For this review, take the finished solid that the model builds, in its own axes (mm). Face numbers are marked on the shaded views. A direction names the side the tool comes from. Coordinates: 2 decimals unless noted, no trailing zeros. Write each loop counter-clockwise with the first axis right and the second up, starting at its lowest first coordinate (ties: lowest second). Pieces come first, ordered by that corner, then holes. Notation, with made-up numbers: M 55,58.25 L 109,58.25 A17 ccw 109,85.25 Z; hole C 21.25,-29 d9. An arc over 180 degrees is marked long. Return JSON: item names as keys, results as strings.
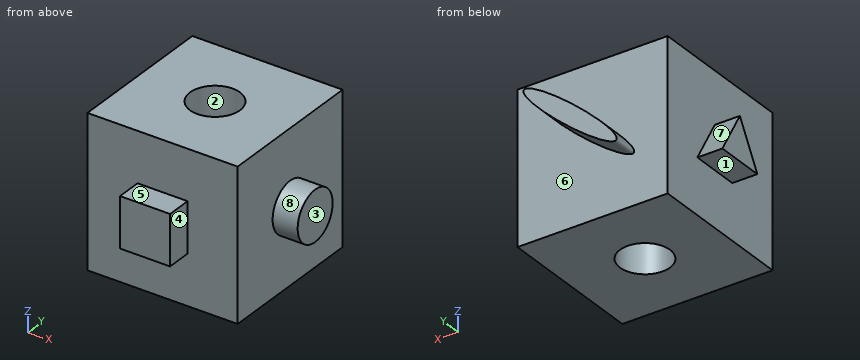
```python
from build123d import *

# Parameters (mm, degrees)
F0_W      = 76.2
F0_H      = 76.2
F1_DEPTH  = 76.2
F2_W      = 25.4
F2_H      = 25.4
F3_DEPTH  = 12.7
F4_R      = 12.7
F5_DEPTH  = 12.7
F7_D      = 25.4
F9_DEPTH  = 12.7
F11_DEPTH = 12.7


with BuildPart() as f1:
    # F0 (on Front) → F1 (new body)
    with BuildSketch(Plane.XZ):
        with Locations((-25.095452, 28.064179)):
            Rectangle(F0_W, F0_H)
    extrude(amount=F1_DEPTH)

    # F2 (on face) → F3 (join)
    with BuildSketch(Plane.XZ.offset(76.2)):
        with Locations((-25.095452, 28.064179)):
            Rectangle(F2_W, F2_H)
    extrude(amount=F3_DEPTH)

    # F4 (on face) → F5 (join)
    with BuildSketch(Plane.YZ.offset(13.004548)):
        with Locations((-38.1, 28.064179)):
            Circle(F4_R)
    extrude(amount=F5_DEPTH)

    # F7 (through all)
    with Locations(Plane.XY.offset(66.164179)):
        with Locations((-25.095452, -38.1)):
            Hole(F7_D / 2)

    # F8 (on face) → F9 (join)
    with BuildSketch(Plane(origin=(-63.195452, 0, 0), x_dir=(0, -1, 0), z_dir=(-1, 0, 0))):
        Polygon((46.956852, 17.904179), (34.256852, 39.901224), (21.556852, 17.904179), align=None)
    extrude(amount=F9_DEPTH)

    # F10 (on face) → F11 (join)
    with BuildSketch(Plane(origin=(0, 0, 0), x_dir=(-1, 0, 0), z_dir=(0, 1, 0))):
        with BuildLine():
            add(Edge.make_bspline(
                [(-0.974158, 55.745363), (-6.054851, 49.801911), (31.750569, 22.627692), (69.555988, -4.546527), (36.831261, 28.571144), (4.106534, 61.688816), (-0.974158, 55.745363)],
                knots=[0, 0, 0, 2.094395, 2.094395, 4.18879, 4.18879, 6.283185, 6.283185, 6.283185], degree=2, weights=[1, 0.5, 1, 0.5, 1, 0.5, 1]))
        make_face()
    extrude(amount=F11_DEPTH)


solid = f1.part
```
1. For the marked faces 4, 5, 6, 7 and 8, list the 3-axis set-ups (+Z, -Z, +X, -X, +Y, -Y) from which the entire face can be reached by the end or side of a thin tool; tool diameter is ignored.
Checks:
{"face 4": "+Z, -Z, +X, -Y", "face 5": "+Z, +X, -X, -Y", "face 6": "+Y", "face 7": "+Z, -X, +Y", "face 8": "+X"}
2. Clearance check with flat-ended pins moving along their axes: pin 1 Ø2 at (y, z) = (-8, 39) entering from +X; pin 2 Ø6.5 at (x, y) = (-19.5, -83.5) entering from -Z; pin 3 Ø10 at (x, y) = (-68.5, -35) entering from -Z. State where each tip first meets the part, or that it passes through.
Checks:
{"pin 1": "x = 13", "pin 2": "z = 15.36", "pin 3": "z = 17.9"}
3. Wall thickness on L1, parallel to X at y = -38, z = 8; L2, parallel to X at y = -1, z = -6; L3, parallel to Y at x = -26, z = 58.5: over which ranges is each line inside the solid? List them lowest first. Write a range as from..to.
Checks:
{"L1": "-63.2..-37.8, -12.4..13", "L2": "-63.2..13", "L3": "-76.2..-50.77, -25.43..0"}
4. We need section D-D (y = -73.5). State the section outline as (x, z) points, plus the area to 3 significant figures.
Checks:
{"outline": "M -63.2,-10.04 L 13,-10.04 L 13,66.16 L -63.2,66.16 Z", "area": "5,810 mm2"}
5. Draft analysis for pull direction X (two halves, no side actions). For the marked faces 1, 2 and 3, state which applies: +X half, -X half, draft (parallel to the pull), parting line (faces both ways), or undercut.
Checks:
{"face 1": "draft", "face 2": "undercut", "face 3": "+X half"}
6. We need section A-A (y = -39.5). State the section outline as (x, z) points.
Checks:
{"outline": "M -75.9,17.9 L -63.2,17.9 L -63.2,-10.04 L -37.72,-10.04 L -37.72,66.16 L -63.2,66.16 L -63.2,30.82 L -75.9,30.82 Z; M -12.47,-10.04 L 13,-10.04 L 13,15.44 L 25.7,15.44 L 25.7,40.69 L 13,40.69 L 13,66.16 L -12.47,66.16 Z"}
7. We need section B-B (z = -2). State the section outline as (x, y) points.
Checks:
{"outline": "M -63.2,-76.2 L 13,-76.2 L 13,0 L -63.2,0 Z; hole C -25.1,-38.1 d25.4"}
8. We need section C-C (x = 10.5). State the section outline as (y, z) points.
Checks:
{"outline": "M -76.2,-10.04 L 0,-10.04 L 0,66.16 L -76.2,66.16 Z"}
